Work out the finished part from the listing and answer in its coordinate system (mm). Face numbers are marked on the shaded views. A direction names the side the tool comes from. Give positions to 0.01 mm unless a question says otherwise; leave off trailing zeros. Loops run counter-clockwise (first coordinate to the right, second up) from the corner with the lowest first, then second, coordinate; pieces in that order, holes last. Notation, with made-up numbers: (-11.75, -34) - (17.25, -34) arc R28 cw to (17.25, 2) - close; hole circle Ø11 at (66.5, -38.75). An arc over 180 degrees is marked (long way). One line per item, written item: value.
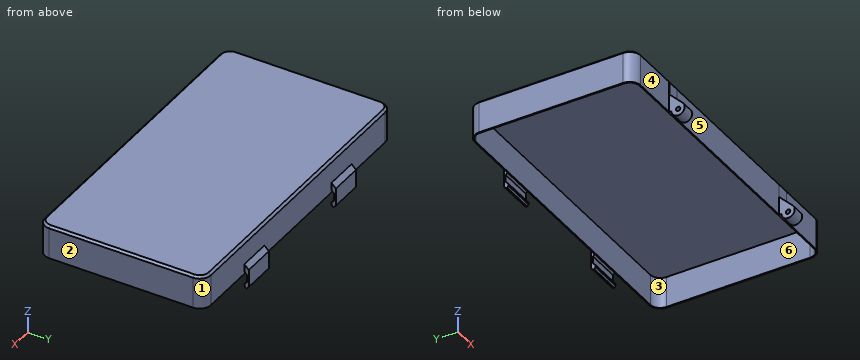
from build123d import *

# Parameters (mm, degrees)
PAD002_DEPTH         = 15
POCKET002_DEPTH      = 14
SKETCH006_R          = 1
PAD003_DEPTH         = 140
SKETCH007_W          = 26.2
SKETCH007_H          = 10
SKETCH007_W_2        = 76.4
POCKET003_DEPTH      = 18.001
SKETCH011_W          = 15
SKETCH011_H          = 11
PAD005_DEPTH         = 2
POCKET006_DEPTH      = 140.001
POCKET006_DEPTH_BACK = 0.001
CHAMFER_SIZE         = 1


with BuildPart() as part:
    # Sketch004 → Pad002 (new body)
    with BuildSketch(Plane.XY):
        with BuildLine():
            Line((-70, 32.5), (-70, -32.5))
            ThreePointArc((-70, -32.5), (-68.535534, -36.035534), (-65, -37.5))
            Line((-65, -37.5), (65, -37.5))
            ThreePointArc((65, -37.5), (68.535534, -36.035534), (70, -32.5))
            Line((70, -32.5), (70, 32.5))
            ThreePointArc((70, 32.5), (68.535534, 36.035534), (65, 37.5))
            Line((65, 37.5), (-65, 37.5))
            ThreePointArc((-65, 37.5), (-68.535534, 36.035534), (-70, 32.5))
        make_face()
    extrude(amount=PAD002_DEPTH)

    # Sketch005 (on Face9 of Pad002) → Pocket002 (cut)
    with BuildSketch(Plane(origin=(0, 0, 0), x_dir=(1, 0, 0), z_dir=(0, 0, -1))):
        with BuildLine():
            Line((-69.5, 32.5), (-69.5, -32.5))
            ThreePointArc((-69.5, -32.5), (-68.181981, -35.681981), (-65, -37))
            Line((-65, -37), (65, -37))
            ThreePointArc((65, -37), (68.181981, -35.681981), (69.5, -32.5))
            Line((69.5, -32.5), (69.5, 32.5))
            ThreePointArc((69.5, 32.5), (68.181981, 35.681981), (65, 37))
            Line((65, 37), (-65, 37))
            ThreePointArc((-65, 37), (-68.181981, 35.681981), (-69.5, 32.5))
        make_face()
    extrude(amount=-POCKET002_DEPTH, mode=Mode.SUBTRACT)

    # Sketch006 (on Face10 of Pocket002) → Pad003 (join)
    with BuildSketch(Plane.YZ.offset(70)):
        with BuildLine():
            ThreePointArc((-43.62132, 2.12132), (-42.64805, -2.771639), (-38.5, 0))
            Line((-38.5, 0), (-37.5, 0))
            Line((-37.5, 0), (-37.5, 8.242641))
            Line((-43.62132, 2.12132), (-37.5, 8.242641))
        make_face()
        with Locations((-41.5, 0)):
            Circle(SKETCH006_R, mode=Mode.SUBTRACT)
    extrude(amount=-PAD003_DEPTH)

    # Sketch007 (on Face4 of Pad003) → Pocket003 (cut, through all)
    with BuildSketch(Plane.XY.offset(15)):
        with Locations((56.9, -42.49)):
            Rectangle(SKETCH007_W, SKETCH007_H)
        with Locations((0, -42.49)):
            Rectangle(SKETCH007_W_2, SKETCH007_H)
        with Locations((-56.9, -42.49)):
            Rectangle(SKETCH007_W, SKETCH007_H)
    extrude(amount=-POCKET003_DEPTH, mode=Mode.SUBTRACT)

    # Sketch011 (on Face6 of Pocket003) → Pad005 (join)
    with BuildSketch(Plane(origin=(0, 37.5, 0), x_dir=(-1, 0, 0), z_dir=(0, 1, 0))):
        with Locations((32.5, -1)):
            Rectangle(SKETCH011_W, SKETCH011_H)
        with Locations((-32.5, -1)):
            Rectangle(SKETCH011_W, SKETCH011_H)
    extrude(amount=PAD005_DEPTH)

    # Sketch012 (on Face1 of Pad005) → Pocket006 (cut, two sides)
    with BuildSketch(Plane(origin=(-70, 0, 0), x_dir=(0, -1, 0), z_dir=(-1, 0, 0))) as pocket006_sk:
        Polygon((-38.5, -6.5), (-39.5, -5.5), (-39.5, -6.5), align=None)
        Polygon((-37.5, 4.5), (-39.5, 2.5), (-39.5, 4.5), align=None)
        Polygon((-37.5, 1), (-38.7, -0.2), (-38.7, -3.5), (-37.5, -4.7), align=None)
        Polygon((-37.5, -5.633975), (-38, -6.5), (-37.5, -6.5), align=None)
    extrude(amount=-POCKET006_DEPTH, mode=Mode.SUBTRACT)
    extrude(pocket006_sk.sketch, amount=POCKET006_DEPTH_BACK, mode=Mode.SUBTRACT)

    # Chamfer
    chamfer_edges = [part.edges().sort_by_distance(p)[0] for p in [
        (-68.535534, 36.035534, 15),
        (0, 37.5, 15),
        (68.535534, 36.035534, 15),
        (70, 0, 15),
        (68.645569, -35.921962, 15),
        (54.558035, -37.49, 15),
        (43.8, -37.495, 15),
        (41, -37.5, 15),
        (38.2, -37.495, 15),
        (0, -37.49, 15),
        (-38.2, -37.495, 15),
        (-41, -37.5, 15),
        (-43.8, -37.495, 15),
        (-54.558035, -37.49, 15),
        (-68.645569, -35.921962, 15),
        (-70, 0, 15),
    ]]
    chamfer(chamfer_edges, length=CHAMFER_SIZE)


solid = part.part
1. The mould has two halves that part along Y. Classify the marked faces 1, 2 and 3: released by +Y, released by -Y, zero draft, split by the parting line, or undercut.
Output:
face 1: released by +Y
face 2: zero draft
face 3: undercut
2. Section B-B (x = 29.5) is taken. Write down the section's boundary in (y, z), and give its area (3 significant figures).
Output:
outline: (-37.49, 0) - (-37, 0) - (-37, 14) - (37, 14) - (37, 0) - (37.5, 0) - (37.5, 1) - (38.7, -0.2) - (38.7, -3.5) - (37.5, -4.7) - (37.5, -5.63) - (38, -6.5) - (38.5, -6.5) - (39.5, -5.5) - (39.5, 2.5) - (37.5, 4.5) - (37.5, 14) - (36.5, 15) - (-36.49, 15) - (-37.49, 14) - close
area: 102 mm²
3. Find the intervals of material crossed by line 1 along X through (y, z) = (21.5, 2.5); line 2 along Y through (x, z) = (9.5, 12); line 3 along Z through (x, y) = (-18, 13), in increasing order.
Output:
line 1: x = -70 to -69.5, 69.5 to 70
line 2: y = -37.49 to -37, 37 to 37.5
line 3: z = 14 to 15
4. For the marked faces 4, 5 and 6, determine the directions among +Z, -Z, +X, -X, +Y, -Y from which every point of the face is accessible in a straight line to the end or side of a thin tool.
Output:
face 4: +Z, -Z, -X, -Y
face 5: +Z, -Z, -Y
face 6: -Z
5. Flat-ended cylindrical pins translate along their axes: pin 1 Ø7 at (x, z) = (2, 7.5) entering from +Y; pin 2 Ø0.6 at (y, z) = (38.5, 1.5) entering from +X; pin 3 Ø3 at (y, z) = (-41.5, 0) entering from -X. Find the tip coordinate at first contact, or state that the pin passes through.
Output:
pin 1: stops at y = 37.5
pin 2: stops at x = 40
pin 3: stops at x = -43.8
6. Section A-A (x = -53.5) is taken. Write down the section's boundary in (y, z), and give its area (4 significant figures).
Output:
outline: (-37.49, 0) - (-37, 0) - (-37, 14) - (37, 14) - (37, 0) - (37.5, 0) - (37.5, 14) - (36.5, 15) - (-36.49, 15) - (-37.49, 14) - close
area: 87.85 mm²
